```python
from build123d import *

# Parameters (mm, degrees)
SKETCH1_W               = 27
SKETCH1_H               = 6
SKETCH1_R               = 1.6
BOSS_EXTRUDE1_DEPTH     = 8
SKETCH3_W               = 27
SKETCH3_H               = 8
BOSS_EXTRUDE2_DEPTH     = 12
SKETCH2_R               = 1.6
CUT_EXTRUDE1_DEPTH      = 16
CUT_EXTRUDE1_DEPTH_BACK = 4


with BuildPart() as part:
    # Sketch1 → Boss-Extrude1 (new body)
    with BuildSketch(Plane(origin=(0, 0, 0), x_dir=(1, 0, 0), z_dir=(0, 1, 0))):
        with Locations((10, 0)):
            Rectangle(SKETCH1_W, SKETCH1_H)
        Circle(SKETCH1_R, mode=Mode.SUBTRACT)
        with Locations((20, 0)):
            Circle(SKETCH1_R, mode=Mode.SUBTRACT)
    extrude(amount=BOSS_EXTRUDE1_DEPTH)

    # Sketch3 → Boss-Extrude2 (add)
    with BuildSketch(Plane.XY.offset(3)):
        with Locations((10, 4)):
            Rectangle(SKETCH3_W, SKETCH3_H)
    extrude(amount=BOSS_EXTRUDE2_DEPTH)

    # Sketch2 → Cut-Extrude1 (cut, two sides)
    with BuildSketch(Plane.XY) as cut_extrude1_sk:
        with Locations((4.5, 4)):
            Circle(SKETCH2_R)
        with Locations((15.5, 4)):
            Circle(SKETCH2_R)
    extrude(amount=CUT_EXTRUDE1_DEPTH, mode=Mode.SUBTRACT)
    extrude(cut_extrude1_sk.sketch, amount=-CUT_EXTRUDE1_DEPTH_BACK, mode=Mode.SUBTRACT)


solid = part.part
```
Source: CAD feature listing. Evaluate the final solid. Frame: model axes, mm. Coordinates: 2 decimals unless noted, no trailing zeros. Write each loop counter-clockwise with the first axis right and the second up, starting at its lowest first coordinate (ties: lowest second). Pieces come first, ordered by that corner, then holes. Notation, with made-up numbers: (71, 42) -> (82, 42) arc R26 ccw to (82, 77) -> close; hole circle Ø11 at (1.5, 5). An arc over 180 degrees is marked (long way). Return JSON: item names as keys, results as strings. Group by question number.
1) Section query D-D, the plane x = 4.5. Return loops of the section in (y, z), plus the area to 3 significant figures.
2) Section query C-C, the plane z = 5.5. Return loops of the section in (x, y).
3) Section query B-B, the plane y = 7.25. Return loops of the section in (x, z), plus the area to 3 significant figures.
4) Section query A-A, the plane x = 20. Return loops of the section in (y, z), plus the area to 3 significant figures.
5) Contact query for a flat-ended pin moving along its axis: P1, Ø4, axis at x = 4.5, y = 4, coming from the -Z side. Output: stop coordinate, or through.
6) Ray query, line 1 along X through (y, z) = (2, 0); line 2 along Y through (x, z) = (15.5, 7.5); line 3 along Z through (x, y) = (20, 5.75). Return the intervals inside material, ascending.
7) Mould query, pull axis Z, two halves, no side actions, for faces 1 (the face through (10, 4, -3)), 2 (the face through (10, 4, 15)), 3 (the face through (10, 8, 6)), 4 (the face through (18.82, 3.94, -1.08)). Classes: +Z half, -Z half, draft (parallel to the pull), parting line (faces both ways), or undercut.
From the geometry:
{
 "1": {"outline": "(0, -3) -> (2.4, -3) -> (2.4, 15) -> (0, 15) -> close; (5.6, -3) -> (8, -3) -> (8, 15) -> (5.6, 15) -> close", "area": "86.4 mm²"},
 "2": {"outline": "(-3.5, 0) -> (23.5, 0) -> (23.5, 8) -> (-3.5, 8) -> close; hole circle Ø3.2 at (4.5, 4); hole circle Ø3.2 at (15.5, 4)"},
 "3": {"outline": "(-3.5, -3) -> (23.5, -3) -> (23.5, 15) -> (-3.5, 15) -> close; hole circle Ø3.2 at (0, 0); hole circle Ø3.2 at (20, 0)", "area": "470 mm²"},
 "4": {"outline": "(0, -3) -> (8, -3) -> (8, -1.6) -> (0, -1.6) -> close; (0, 1.6) -> (8, 1.6) -> (8, 15) -> (0, 15) -> close", "area": "118 mm²"},
 "5": {"P1": "z = -3"},
 "6": {"line 1": "-3.5 to -1.6, 1.6 to 18.4, 21.6 to 23.5", "line 2": "0 to 2.4, 5.6 to 8", "line 3": "-3 to -1.6, 1.6 to 15"},
 "7": {"face 1": "-Z half", "face 2": "+Z half", "face 3": "draft", "face 4": "undercut"}
}
